from build123d import *

# Parameters (mm, degrees)
SKETCH_1_W          = 62
SKETCH_1_H          = 15
SKETCH_1_R          = 0.9
SKETCH_1_R_2        = 1.5
SKETCH_1_R_3        = 4
EXTRUDE_1_DEPTH     = 2
SKETCH_2_R          = 1.4
EXTRUDE_2_DEPTH     = 2
SKETCH_4_R          = 3
CUT_EXTRUDE_1_DEPTH = 1


with BuildPart() as part:
    # 草图1 → 凸台-拉伸1 (new body)
    # profile 1 of 3: a face of its own
    with BuildSketch(Plane(origin=(0, 0, 0), x_dir=(1, 0, 0), z_dir=(0, 1, 0))):
        Rectangle(SKETCH_1_W, SKETCH_1_H)
        with Locations(Location((-12.330127019, 2.5, 0), (0, 0, 270))):
            Circle(SKETCH_1_R, mode=Mode.SUBTRACT)
        with Locations(Location((24, 3.5, 0), (0, 0, 270))):
            Circle(SKETCH_1_R, mode=Mode.SUBTRACT)
        with Locations(Location((20.5, 0, 0), (0, 0, 270))):
            Circle(SKETCH_1_R, mode=Mode.SUBTRACT)
        with Locations(Location((24, -3.5, 0), (0, 0, 270))):
            Circle(SKETCH_1_R, mode=Mode.SUBTRACT)
        with Locations(Location((27.5, 0, 0), (0, 0, 270))):
            Circle(SKETCH_1_R, mode=Mode.SUBTRACT)
        with Locations(Location((24, 0, 0), (0, 0, 270))):
            Circle(SKETCH_1_R_2, mode=Mode.SUBTRACT)
        with Locations(Location((8, 0, 0), (0, 0, 270))):
            Circle(SKETCH_1_R_3, mode=Mode.SUBTRACT)
        with Locations((-12.330127019, -2.5)):
            Circle(SKETCH_1_R, mode=Mode.SUBTRACT)
        with Locations((-3.669872981, 2.5)):
            Circle(SKETCH_1_R, mode=Mode.SUBTRACT)
        with Locations(Location((-8, 0, 0), (0, 0, 270))):
            Circle(SKETCH_1_R_2, mode=Mode.SUBTRACT)
        with Locations(Location((-3.669872981, -2.5, 0), (0, 0, 270))):
            Circle(SKETCH_1_R, mode=Mode.SUBTRACT)
    # profile 2 of 3: a face of its own
    with BuildSketch(Plane(origin=(0, 0, 0), x_dir=(1, 0, 0), z_dir=(0, 1, 0))):
        with Locations((-12.330127019, -2.5)):
            Circle(SKETCH_1_R)
    # profile 3 of 3: a face of its own
    with BuildSketch(Plane(origin=(0, 0, 0), x_dir=(1, 0, 0), z_dir=(0, 1, 0))):
        with Locations((-3.669872981, 2.5)):
            Circle(SKETCH_1_R)
    extrude(amount=EXTRUDE_1_DEPTH)

    # 草图2 → 凸台-拉伸2 (add)
    with BuildSketch(Plane.XY.offset(7.5)):
        with Locations(Location((-23, 1, 0), (0, 0, 134.415308597))):
            Circle(SKETCH_2_R)
        with Locations(Location((-8, 1, 0), (0, 0, 134.415308597))):
            Circle(SKETCH_2_R)
        with Locations(Location((7, 1, 0), (0, 0, 134.415308597))):
            Circle(SKETCH_2_R)
    extrude(amount=EXTRUDE_2_DEPTH)

    # 草图4 → 切除-拉伸1 (cut)
    with BuildSketch(Plane(origin=(0, 2, 0), x_dir=(1, 0, 0), z_dir=(0, 1, 0))):
        with Locations(Location((-8, 0, 0), (0, 0, 270))):
            Circle(SKETCH_4_R)
    extrude(amount=-CUT_EXTRUDE_1_DEPTH, mode=Mode.SUBTRACT)


solid = part.part
The listing builds one solid part. Answer for the finished solid, in the listing's coordinates (mm). A direction names the side the tool comes from. Round coordinates to 2 decimals unless told otherwise and drop trailing zeros. Loops run counter-clockwise (first coordinate to the right, second up) from the corner with the lowest first, then second, coordinate; pieces in that order, holes last. Notation, with made-up numbers: M 18,72.5 L 32,72.5 A23 ccw 32,83.5 Z; hole C 70,-39 d7. An arc over 180 degrees is marked long. Write each question's results on one line, items separated by ' | '. Start each with the question number.
1) Straight lines are drawn through the part: probe 1 along X at (y, z) = (1.4, 0); probe 2 along X at (y, z) = (1.2, 1.25); probe 3 along X at (y, z) = (1.25, 1.75). For each, find the intervals that lie inside material, in ascending order.
2) Which of the six approach directions +Z, -Z, +X, -X, +Y, -Y give full straight-line access (tool end or side, diameter ignored) to faces 5 (the cylindrical face through (5.63, 0.71, 8.49)), 6 (the cylindrical face through (25.487, 0.986, -0.195)), 7 (the flat face through (0, 2, 0))?
3) Find section D-D on x = -8. Write down the section's boundary in (y, z), plus the area to 3 significant figures.
4) Find section B-B on z = -0.25. Write down the section's boundary in (x, y), plus the area to 3 significant figures.
5) Find section A-A on x = 27.5. Write down the section's boundary in (y, z), plus the area to 3 significant figures.
6) Find section C-C on x = -23. Write down the section's boundary in (y, z).
7) Determine the mould class of faces 1 (the cylindrical face through (-2.91, 0.99, 2.98)), 2 (the flat face through (-31, 1, 0)), 3 (the flat face through (7, 1, 9.5)), 4 (the flat face through (31, 1, 0)) for opening direction X: pulls with the +X half, pulls with the -X half, needs draft (parallel to the pull), parting line crosses it, or undercut.
8) Each of these flat-tipped pins is pushed along its axis until it touches: pin 1 (5 mm diameter, centred on x = -8, z = 0, fed in from -Y); pin 2 (1.6 mm diameter, centred on x = -26.5, y = 1.5, fed in from +Z); pin 3 (3 mm diameter, centred on x = 24, z = 3.5, fed in from +Y). Where does it stop, or does it pass through?
Final values:
1) probe 1: -31 to -11, -5 to 4, 12 to 19.6, 21.4 to 22.5, 25.5 to 26.6, 28.4 to 31 | probe 2: -31 to -10.73, -5.27 to 4.2, 11.8 to 23.17, 24.83 to 31 | probe 3: -31 to -10.44, -5.56 to -4.17, -3.17 to 4.4, 11.6 to 31
2) face 5: +Z | face 6: +Y, -Y | face 7: -Z, +X, -X, +Y
3) outline: M -0.4,7.5 L 0,7.5 L 0,1.5 L 1,1.5 L 1,3 L 2,3 L 2,7.5 L 2.4,7.5 L 2.4,9.5 L -0.4,9.5 Z; M 0,-7.5 L 2,-7.5 L 2,-3 L 1,-3 L 1,-1.5 L 0,-1.5 Z | area: 26.6 mm²
4) outline: M -31,0 L -9.48,0 L -9.48,1 L -10.99,1 L -10.99,2 L -31,2 Z; M -6.52,0 L 4.01,0 L 4.01,2 L -5.01,2 L -5.01,1 L -6.52,1 Z; M 11.99,0 L 19.64,0 L 19.64,2 L 11.99,2 Z; M 21.36,0 L 22.52,0 L 22.52,2 L 21.36,2 Z; M 25.48,0 L 26.64,0 L 26.64,2 L 25.48,2 Z; M 28.36,0 L 31,0 L 31,2 L 28.36,2 Z | area: 86.3 mm²
5) outline: M 0,-7.5 L 2,-7.5 L 2,-0.9 L 0,-0.9 Z; M 0,0.9 L 2,0.9 L 2,7.5 L 0,7.5 Z | area: 26.4 mm²
6) outline: M -0.4,7.5 L 0,7.5 L 0,-7.5 L 2,-7.5 L 2,7.5 L 2.4,7.5 L 2.4,9.5 L -0.4,9.5 Z
7) face 1: undercut | face 2: pulls with the -X half | face 3: needs draft | face 4: pulls with the +X half
8) pin 1: y = 0 | pin 2: z = 7.5 | pin 3: y = 2
